Verification items for the finished model (mm, model axes). A direction names the side the tool comes from. Give positions to 0.01 mm unless a question says otherwise; leave off trailing zeros. Write each loop counter-clockwise with the first axis right and the second up, starting at its lowest first coordinate (ties: lowest second). Pieces come first, ordered by that corner, then holes. Notation, with made-up numbers: (10.5, 13) -> (36.5, 13) arc R35 cw to (36.5, 51) -> close; hole circle Ø9 at (23, -26). An arc over 180 degrees is marked (long way). Write item = value, one per line.
from build123d import *

# Parameters (mm, degrees)
F0_W      = 38
F0_H      = 22
F1_DEPTH  = 20
F2_W      = 38
F2_H      = 22
F3_DEPTH  = 5
F4_R      = 2.5
F5_DEPTH  = 5
F6_R      = 7.5
F6_R_2    = 2.5
F7_DEPTH  = 3
F8_W      = 11
F8_H      = 20
F9_DEPTH  = 1.7
F11_DEPTH = 3
F12_R     = 3
F13_R     = 3


with BuildPart() as f1:
    # F0 (on Top) → F1 (new body)
    with BuildSketch(Plane.XY):
        Rectangle(F0_W, F0_H)
        with BuildLine():
            ThreePointArc((-16.75, 7.3), (-16.1642135624, 8.7142135624), (-14.75, 9.3))
            Line((-14.75, 9.3), (14.75, 9.3))
            ThreePointArc((14.75, 9.3), (16.1642135624, 8.7142135624), (16.75, 7.3))
            Line((16.75, 7.3), (16.75, -7.3))
            ThreePointArc((16.75, -7.3), (16.1642135624, -8.7142135624), (14.75, -9.3))
            Line((14.75, -9.3), (-14.75, -9.3))
            ThreePointArc((-14.75, -9.3), (-16.1642135624, -8.7142135624), (-16.75, -7.3))
            Line((-16.75, -7.3), (-16.75, 7.3))
        make_face(mode=Mode.SUBTRACT)
    extrude(amount=F1_DEPTH)

    # F2 (on face) → F3 (join)
    with BuildSketch(Plane.XY.offset(20)):
        Rectangle(F2_W, F2_H)
    extrude(amount=F3_DEPTH)

    # F4 (on face) → F5 (cut, through all)
    with BuildSketch(Plane(origin=(0, 0, 20), x_dir=(1, 0, 0), z_dir=(0, 0, -1))):
        with BuildLine():
            ThreePointArc((-16.75, 6.05), (-13.5, 2.8), (-10.25, 6.05))
            ThreePointArc((-10.25, 6.05), (-11.2019029611, 8.3480970389), (-13.5, 9.3))
            ThreePointArc((-13.5, 9.3), (-15.7980970389, 8.3480970389), (-16.75, 6.05))
        make_face()
        Circle(F4_R)
    extrude(amount=-F5_DEPTH, mode=Mode.SUBTRACT)

    # F6 (on face) → F7 (cut)
    with BuildSketch(Plane.XY.offset(25)):
        Circle(F6_R)
        Circle(F6_R_2, mode=Mode.SUBTRACT)
    extrude(amount=-F7_DEPTH, mode=Mode.SUBTRACT)

    # F8 (on face) → F9 (cut, through all)
    with BuildSketch(Plane(origin=(0, -9.3, 0), x_dir=(-1, 0, 0), z_dir=(0, 1, 0))):
        with Locations((-5.5, 10)):
            Rectangle(F8_W, F8_H)
    extrude(amount=-F9_DEPTH, mode=Mode.SUBTRACT)

    # F10 (on face) → F11 (cut, through all)
    with BuildSketch(Plane.XY.offset(25)):
        with BuildLine():
            Line((-7.2929760729, 1.75), (-19, 1.75))
            Line((-19, 1.75), (-19, -1.75))
            Line((-19, -1.75), (-7.2929760729, -1.75))
            ThreePointArc((-7.2929760729, -1.75), (-7.5, 0), (-7.2929760729, 1.75))
        make_face()
    extrude(amount=-F11_DEPTH, mode=Mode.SUBTRACT)

    # F12
    f12_edges = [f1.edges().sort_by_distance(p)[0] for p in [
        (-19, -11, 12.5),
        (19, -11, 12.5),
        (19, 11, 12.5),
        (-19, 11, 12.5),
    ]]
    fillet(f12_edges, radius=F12_R)

    # F13
    f13_edges = [f1.edges().sort_by_distance(p)[0] for p in [
        (0, -10.15, 20),
        (11, -10.15, 20),
    ]]
    fillet(f13_edges, radius=F13_R)


solid = f1.part
Item 1: Sectioned sample at D-D on x = -9.5. Record the cut outline in (y, z).
Response values:
outline = (-11, 0) -> (-9.3, 0) -> (-9.3, 20) -> (9.3, 20) -> (9.3, 0) -> (11, 0) -> (11, 25) -> (1.75, 25) -> (1.75, 22) -> (-1.75, 22) -> (-1.75, 25) -> (-11, 25) -> close
Item 2: Set-up check for faces 4 (the flat face through (11, -10, 8)), 5 (the cylindrical face through (-0.54, 2.44, 20.99)), 6 (the flat face through (-13, -1.75, 24)), 7 (the cylindrical face through (7.494, -0.305, 23.521)), 8 (the cylindrical face through (16.18, -8.7, 9.86)): record each of +Z, -Z, +X, -X, +Y, -Y from which the full face is reachable in a straight line by a thin tool's end or side.
Response values:
face_4 = -Z, -Y
face_5 = +Z, -Z
face_6 = +Z, -X
face_7 = +Z
face_8 = -Z
Item 3: Mould release check, pull along Y, two halves, no side actions. Record for faces 1 (the flat face through (-13, 1.75, 24)), 2 (the flat face through (0, -10, 8)), 3 (the flat face through (0, 11, 12)): +Y half, -Y half, draft (parallel to the pull), parting line (faces both ways), or undercut.
Response values:
face_1 = undercut
face_2 = draft
face_3 = +Y half
Item 4: Sectioned sample at B-B on z = 14. Record the cut outline in (x, y).
Response values:
outline = (-19, -8) arc R3 ccw to (-16, -11) -> (0, -11) -> (0, -9.3) -> (-14.75, -9.3) arc R2 cw to (-16.75, -7.3) -> (-16.75, 7.3) arc R2 cw to (-14.75, 9.3) -> (14.75, 9.3) arc R2 cw to (16.75, 7.3) -> (16.75, -7.3) arc R2 cw to (14.75, -9.3) -> (11, -9.3) -> (11, -11) -> (16, -11) arc R3 ccw to (19, -8) -> (19, 8) arc R3 ccw to (16, 11) -> (-16, 11) arc R3 ccw to (-19, 8) -> close
Item 5: Sectioned sample at A-A on y = 0. Record the cut outline in (x, z), then the cut area to 4 significant figures.
Response values:
outline = (-19, 0) -> (-16.75, 0) -> (-16.75, 20) -> (-2.5, 20) -> (-2.5, 22) -> (-19, 22) -> close; (2.5, 20) -> (16.75, 20) -> (16.75, 0) -> (19, 0) -> (19, 25) -> (7.5, 25) -> (7.5, 22) -> (2.5, 22) -> close
area = 190.5 mm^2
Item 6: Material ranges on line 1 (X direction, y = 1, z = 9.5); line 2 (Y direction, x = 0, z = 20.8); line 3 (X direction, y = 0, z = 20.6), recorded low to high.
Response values:
line_1 = -19 to -16.75, 16.75 to 19
line_2 = -11 to -2.5, 2.5 to 11
line_3 = -19 to -2.5, 2.5 to 19
Item 7: Go/stop test with flat-tipped pins: P1, Ø4.5, axis at x = -11, y = -0.5, coming from the +Z side; P2, Ø6, axis at x = 5.5, y = 1, coming from the -Z side; P3, Ø0.5, axis at y = -10, z = 8, coming from the -X side; P4, Ø1.9, axis at y = -10.5, z = 9.5, coming from the +X side. Record where each tip stops, or that it passes through.
Response values:
P1 = 25
P2 = 20
P3 = -18.44
P4 = 18.57
